Input: part model. Units: mm. Frame: model coordinates. Face numbers are marked on the shaded views. A direction names the side the tool comes from. Round coordinates to 2 decimals unless told otherwise and drop trailing zeros. Loops run counter-clockwise (first coordinate to the right, second up) from the corner with the lowest first, then second, coordinate; pieces in that order, holes last. Notation, with made-up numbers: (75, 33) -> (130, 33) arc R29 ccw to (130, 67) -> close; hole circle Ø11 at (59, 23). An arc over 180 degrees is marked (long way). Answer as a JSON object with one key per item and string values.
Autodesk Inventor part; units mm, degrees
ref_plane "YZ Plane" through (0, 0, 0) normal (1, 0, 0) x (0, 1, 0)
ref_plane "XZ Plane" through (0, 0, 0) normal (0, 1, 0) x (-1, 0, 0)
ref_plane "XY Plane" through (0, 0, 0) normal (0, 0, 1) x (1, 0, 0)
sketch "Sketch1" plane through (0, 0, 0) normal (0, 0, 1) x (1, 0, 0)
  arc A0 (-8.2061, -3.1475) -> (-7.8618, -4.0207) centre (-7.8531, -3.5128) ccw
  line L0 (-0.8184, 3.9914) -> (-8.2061, -3.1475)
  arc A1 (-0.4592, 4.1402) -> (-0.8184, 3.9914) centre (-0.4592, 3.6322) ccw
  line L1 (0.4145, 4.1402) -> (-0.4592, 4.1402)
  arc A2 (0.8488, 3.962) -> (0.4145, 4.1402) centre (0.4606, 3.6343) ccw
  line L2 (8.2061, -3.1475) -> (0.8488, 3.962)
  arc A3 (7.8618, -4.0207) -> (8.2061, -3.1475) centre (7.8531, -3.5128) ccw
  line L3 (-7.8618, -4.0207) -> (7.8618, -4.0207)
  circle A4 centre (21.4376, -2.3876) radius 2.032
  circle A5 centre (-21.4376, -2.3876) radius 2.032
  arc A6 (16.9463, 6.35) -> (15.8972, 5.301) centre (16.9463, 5.301) ccw
  line L4 (15.8972, 5.301) -> (15.8972, 5.1892)
  arc A7 (15.8972, 5.1892) -> (16.9463, 4.1402) centre (16.9463, 5.1892) ccw
  line L5 (16.9463, 4.1402) -> (19.0952, 4.1402)
  arc A8 (19.8159, 2.3571) -> (19.0952, 4.1402) centre (19.0952, 3.103) ccw
  line L6 (19.8159, 2.3571) -> (16.5346, -0.8136)
  arc A9 (14.3374, -1.7018) -> (16.5346, -0.8136) centre (14.3374, 1.4602) ccw
  line L7 (14.3374, -1.7018) -> (11.0626, -1.7018)
  arc A10 (8.8654, -0.8136) -> (11.0626, -1.7018) centre (11.0626, 1.4602) ccw
  line L8 (8.8654, -0.8136) -> (5.5841, 2.3571)
  arc A11 (6.3048, 4.1402) -> (5.5841, 2.3571) centre (6.3048, 3.103) ccw
  line L9 (6.3048, 4.1402) -> (8.4349, 4.1402)
  arc A12 (8.4349, 4.1402) -> (9.4839, 5.1892) centre (8.4349, 5.1892) ccw
  line L10 (9.4839, 5.1892) -> (9.4839, 5.301)
  arc A13 (9.4839, 5.301) -> (8.4349, 6.35) centre (8.4349, 5.301) ccw
  line L11 (8.4349, 6.35) -> (7.3479, 6.35)
  arc A14 (6.332, 6.35) -> (7.3479, 6.35) centre (6.8399, 6.3541) ccw
  line L12 (6.332, 6.35) -> (3.1719, 6.35)
  arc A15 (2.156, 6.35) -> (3.1719, 6.35) centre (2.6639, 6.3541) ccw
  line L13 (2.156, 6.35) -> (-2.156, 6.35)
  arc A16 (-3.1719, 6.35) -> (-2.156, 6.35) centre (-2.6639, 6.3541) ccw
  line L14 (-3.1719, 6.35) -> (-6.3893, 6.35)
  arc A17 (-7.4052, 6.35) -> (-6.3893, 6.35) centre (-6.8973, 6.3541) ccw
  line L15 (-7.4052, 6.35) -> (-8.4349, 6.35)
  arc A18 (-8.4349, 6.35) -> (-9.4839, 5.301) centre (-8.4349, 5.301) ccw
  line L16 (-9.4839, 5.301) -> (-9.4839, 5.1892)
  arc A19 (-9.4839, 5.1892) -> (-8.4349, 4.1402) centre (-8.4349, 5.1892) ccw
  line L17 (-8.4349, 4.1402) -> (-6.3048, 4.1402)
  arc A20 (-5.5841, 2.3571) -> (-6.3048, 4.1402) centre (-6.3048, 3.103) ccw
  line L18 (-5.5841, 2.3571) -> (-8.8654, -0.8136)
  arc A21 (-11.0626, -1.7018) -> (-8.8654, -0.8136) centre (-11.0626, 1.4602) ccw
  line L19 (-11.0626, -1.7018) -> (-14.3374, -1.7018)
  arc A22 (-16.5346, -0.8136) -> (-14.3374, -1.7018) centre (-14.3374, 1.4602) ccw
  line L20 (-16.5346, -0.8136) -> (-19.809, 2.3504)
  arc A23 (-19.0855, 4.1402) -> (-19.809, 2.3504) centre (-19.0855, 3.0991) ccw
  line L21 (-19.0855, 4.1402) -> (-17.0099, 4.1402)
  arc A24 (-17.0099, 4.1402) -> (-15.9609, 5.1892) centre (-17.0099, 5.1892) ccw
  line L22 (-15.9609, 5.1892) -> (-15.9609, 5.301)
  arc A25 (-15.9609, 5.301) -> (-17.0099, 6.35) centre (-17.0099, 5.301) ccw
  line L23 (-17.0099, 6.35) -> (-18.0395, 6.35)
  arc A26 (-19.0555, 6.35) -> (-18.0395, 6.35) centre (-18.5475, 6.3541) ccw
  line L24 (-19.0555, 6.35) -> (-22.2504, 6.35)
  arc A27 (-23.2664, 6.354) -> (-22.2504, 6.35) centre (-22.7584, 6.3541) ccw
  arc A28 (-23.2664, 6.354) -> (-25.4, 4.2459) centre (-23.2918, 4.2459) ccw
  line L25 (-25.4, 4.2459) -> (-25.4, -4.2459)
  arc A29 (-25.4, -4.2459) -> (-23.2881, -6.4371) centre (-23.2933, -4.3288) ccw
  arc A30 (-22.2765, -6.35) -> (-23.2881, -6.4371) centre (-22.7808, -6.4114) ccw
  line L26 (-22.2765, -6.35) -> (-19.0448, -6.35)
  arc A31 (-18.0363, -6.35) -> (-19.0448, -6.35) centre (-18.5406, -6.4114) ccw
  line L27 (-18.0363, -6.35) -> (-7.4084, -6.35)
  arc A32 (-6.3999, -6.35) -> (-7.4084, -6.35) centre (-6.9041, -6.4114) ccw
  line L28 (-6.3999, -6.35) -> (-3.1684, -6.35)
  arc A33 (-2.1599, -6.35) -> (-3.1684, -6.35) centre (-2.6641, -6.4114) ccw
  line L29 (-2.1599, -6.35) -> (2.1135, -6.35)
  arc A34 (3.122, -6.35) -> (2.1135, -6.35) centre (2.6177, -6.4114) ccw
  line L30 (3.122, -6.35) -> (6.3882, -6.35)
  arc A35 (7.3967, -6.35) -> (6.3882, -6.35) centre (6.8925, -6.4114) ccw
  line L31 (7.3967, -6.35) -> (18.0231, -6.35)
  arc A36 (19.0317, -6.35) -> (18.0231, -6.35) centre (18.5274, -6.4114) ccw
  line L32 (19.0317, -6.35) -> (22.2866, -6.35)
  arc A37 (23.2982, -6.4371) -> (22.2866, -6.35) centre (22.7909, -6.4114) ccw
  arc A38 (23.2982, -6.4371) -> (25.4, -4.2459) centre (23.2933, -4.3288) ccw
  line L33 (25.4, -4.2459) -> (25.4, 4.2355)
  arc A39 (25.4, 4.2355) -> (23.2665, 6.354) centre (23.2918, 4.2459) ccw
  arc A40 (22.2505, 6.35) -> (23.2665, 6.354) centre (22.7585, 6.3541) ccw
  line L34 (22.2505, 6.35) -> (18.998, 6.35)
  arc A41 (17.9823, 6.35) -> (18.998, 6.35) centre (18.4902, 6.3374) ccw
  line L35 (17.9823, 6.35) -> (16.9463, 6.35)
  point P0 (0, 0)
extrude "Extrusion1" add sketch "Sketch1" against normal blind 50.8
properties part number "2012_2in"
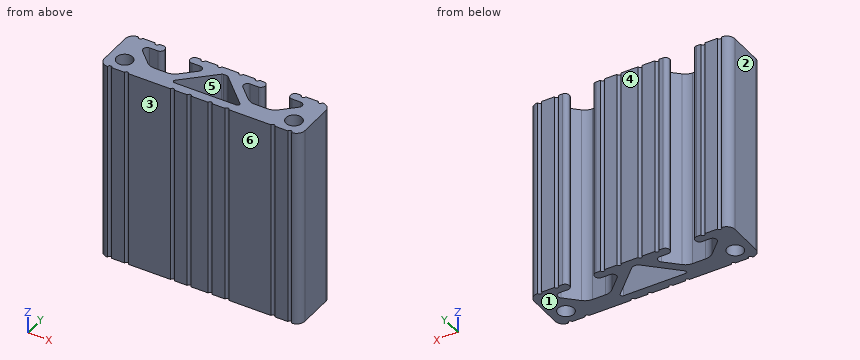
1) Contact query for flat-ended pins moving along their axis: P1, Ø1.6, axis at x = -20.5, z = -22, coming from the +Y side; P2, Ø1, axis at x = -5.5, z = -27, coming from the -Y side; P3, Ø6.5, axis at x = 21.44, y = -2.39, coming from the -Z side; P4, Ø1.6, axis at x = 12.5, z = -26, coming from the +Y side. Output: stop coordinate, or through.
Output:
{"P1": "stops at y = 6.35", "P2": "stops at y = -6.35", "P3": "stops at z = -50.8", "P4": "stops at y = -1.7"}
2) Reachability of the marked faces 4, 5 and 6 from +Z, -Z, +X, -X, +Y, -Y: full face, straight path, thin tool, end or side. Return the list, or none.
Output:
{"face 4": "+Z, -Z, +X, -X, +Y", "face 5": "+Z, -Z", "face 6": "+Z, -Z, -Y"}
3) Section A-A, the plane x = -21. Output: boundary loops of the cut face in (y, z), plus the area to 3 significant figures.
Output:
{"outline": "(-6.35, -50.8) -> (-4.37, -50.8) -> (-4.37, 0) -> (-6.35, 0) -> close; (-0.4, -50.8) -> (6.35, -50.8) -> (6.35, 0) -> (-0.4, 0) -> close", "area": "444 mm^2"}
4) Section B-B, the plane y = 3. Output: boundary loops of the cut face in (x, z).
Output:
{"outline": "(-25.4, -50.8) -> (-20.12, -50.8) -> (-20.12, 0) -> (-25.4, 0) -> close; (-5.27, -50.8) -> (-1.84, -50.8) -> (-1.84, 0) -> (-5.27, 0) -> close; (1.84, -50.8) -> (5.27, -50.8) -> (5.27, 0) -> (1.84, 0) -> close; (20.13, -50.8) -> (25.4, -50.8) -> (25.4, 0) -> (20.13, 0) -> close"}
5) Ray query, probe 1 along Y at (x, z) = (21.5, -37); probe 2 along X at (y, z) = (3.75, -27); probe 3 along X at (y, z) = (-3.75, -13.5). Return the intervals inside material, ascending.
Output:
{"probe 1": "y = -6.35 to -4.42, -0.36 to 6.35", "probe 2": "x = -25.4 to -19.9, -5.49 to -1.07, 1.07 to 5.49, 19.91 to 25.4", "probe 3": "x = -25.4 to -22.95, -19.93 to -8.3, 8.3 to 19.93, 22.95 to 25.4"}
6) Section C-C, the plane x = -13. Output: boundary loops of the cut face in (y, z), plus the area to 3 significant figures.
Output:
{"outline": "(-6.35, -50.8) -> (-1.7, -50.8) -> (-1.7, 0) -> (-6.35, 0) -> close", "area": "236 mm^2"}
7) Draft query along X for the marked faces 1, 2 and 3. Return one class per face: +X half, -X half, draft (parallel to the pull), parting line (faces both ways), or undercut.
Output:
{"face 1": "draft", "face 2": "-X half", "face 3": "undercut"}
8) Section D-D, the plane z = -38.5. Count the separate pieces of the cut face and the enclosed holes in it, plus the area to 3 significant figures.
Output:
{"separate pieces": "1", "enclosed holes": "3", "area": "368 mm^2"}
